Geometry: final body of the model. Coordinates: model frame, mm. A direction names the side the tool comes from. Give positions to 0.01 mm unless a question says otherwise; leave off trailing zeros. Loops run counter-clockwise (first coordinate to the right, second up) from the corner with the lowest first, then second, coordinate; pieces in that order, holes last.
from build123d import *

# Parameters (mm, degrees)
F1_DEPTH  = 22.352
F2_DEPTH  = 3.175
F3_R      = 10.922
F5_DEPTH  = 9.652
F6_DEPTH  = 25.4
F7_R      = 3.175
F9_DEPTH  = 9.652
F8_R      = 6.35
F10_DEPTH = 3.175


with BuildPart() as f1:
    # F0 (on Front) → F1 (new body, symmetric)
    with BuildSketch(Plane.XZ):
        Polygon((28.1862923991, 4.826), (2.7862923991, 4.826), (-16.2637076009, 37.8215678842), (-24.6225847982, 32.9955678842), (-2.7862923991, -4.826), (63.5, -4.826), (63.5, 4.826), align=None)
    extrude(amount=F1_DEPTH, both=True)

    # F0 (on Front) → F2 (join, symmetric)
    with BuildSketch(Plane.XZ):
        Polygon((-16.2637076009, 37.8215678842), (2.7862923991, 4.826), (28.1862923991, 4.826), align=None)
    extrude(amount=F2_DEPTH, both=True)

    # F3
    f3_edges = [f1.edges().sort_by_distance(p)[0] for p in [
        (-20.443146, -22.352, 35.408568),
        (-20.443146, 22.352, 35.408568),
    ]]
    fillet(f3_edges, radius=F3_R)

    # F4 (on face) → F5 (join)
    with BuildSketch(Plane.XY.offset(4.826)):
        with BuildLine():
            Line((63.5, -9.652), (63.5, -22.352))
            ThreePointArc((63.5, -22.352), (85.852, 0), (63.5, 22.352))
            Line((63.5, 22.352), (63.5, 9.652))
            Line((63.5, 9.652), (66.2862923991, 9.652))
            ThreePointArc((66.2862923991, 9.652), (75.9382923991, 0), (66.2862923991, -9.652))
            Line((66.2862923991, -9.652), (63.5, -9.652))
        make_face()
    extrude(amount=-F5_DEPTH)

    # F4 (on face) → F6 (cut)
    with BuildSketch(Plane.XY.offset(4.826)):
        with BuildLine():
            Line((40.8862923991, -9.652), (63.5, -9.652))
            Line((63.5, -9.652), (63.5, 9.652))
            Line((63.5, 9.652), (40.8862923991, 9.652))
            ThreePointArc((40.8862923991, 9.652), (31.2342923991, 0), (40.8862923991, -9.652))
        make_face()
    extrude(amount=-F6_DEPTH, mode=Mode.SUBTRACT)

    # F7 (on face) → F9 (cut, through all)
    with BuildSketch(Plane(origin=(-4.1794385987, 0, -2.413), x_dir=(0, -1, 0), z_dir=(-0.8660254038, 0, -0.5))):
        with Locations((11.43, 29.9642923991)):
            Circle(F7_R)
        with BuildLine():
            ThreePointArc((-8.255, 29.9642923991), (-11.43, 33.1392923991), (-14.605, 29.9642923991))
            ThreePointArc((-14.605, 29.9642923991), (-11.43, 26.7892923991), (-8.255, 29.9642923991))
        make_face()
    extrude(amount=-F9_DEPTH, mode=Mode.SUBTRACT)

    # F8 (on face) → F10 (cut)
    with BuildSketch(Plane(origin=(4.1794385987, 0, 2.413), x_dir=(0, 1, 0), z_dir=(0.8660254038, 0, 0.5))):
        with Locations((-11.43, 29.9642923991)):
            Circle(F8_R)
        with Locations((11.43, 29.9642923991)):
            Circle(F8_R)
    extrude(amount=-F10_DEPTH, mode=Mode.SUBTRACT)


solid = f1.part
Item 1: Pin query (flat end, axial travel): pin 1 (2 mm diameter, centred on y = 10, z = 30.5, fed in from +X); pin 2 (1 mm diameter, centred on x = 51, y = -8.5, fed in from +Z); pin 3 (3 mm diameter, centred on x = -13, y = 14, fed in from +Z); pin 4 (10 mm diameter, centred on x = 16, z = 18, fed in from -Y) (3 decimals). Return the tip coordinate at first contact, or that it passes through.
Values follow:
pin 1: stops at x = -15.13
pin 2: passes through
pin 3: stops at z = 34.77
pin 4: stops at y = -3.175
Item 2: Section query A-A on x = 45.5. Return loops of the section in (y, z).
Values follow:
outline: (-22.35, -4.83) - (-9.65, -4.83) - (-9.65, 4.83) - (-22.35, 4.83) - close; (9.65, -4.83) - (22.35, -4.83) - (22.35, 4.83) - (9.65, 4.83) - close
Item 3: Ray query, probe 1 along Y at (x, z) = (47, 2.5); probe 2 along Y at (x, z) = (66.5, 3); probe 3 along Z at (x, y) = (79, 1.5). Return the intervals inside material, ascending.
Values follow:
probe 1: y = -22.35 to -9.65, 9.65 to 22.35
probe 2: y = -22.15 to -9.65, 9.65 to 22.15
probe 3: z = -4.83 to 4.83
Item 4: Set-up query: faces 1 (the face through (-12.186, -8.697, 24.408)), 2 (the face through (6, -3.175, 15)), 3 (the face through (53, -9.652, 0)). Return all of +Z, -Z, +X, -X, +Y, -Y with unobstructed straight access to the full face (end or side cutting, diameter ignored); none if empty.
Values follow:
face 1: none
face 2: +Z, +X, -Y
face 3: +Z, -Z
Item 5: Section query B-B on y = 0. Return loops of the section in (x, z), plus the area to 3 significant figures.
Values follow:
outline: (-24.62, 33) - (-2.79, -4.83) - (31.23, -4.83) - (31.23, 4.83) - (28.19, 4.83) - (-16.26, 37.82) - close; (75.94, -4.83) - (85.85, -4.83) - (85.85, 4.83) - (75.94, 4.83) - close
area: 1,210 mm2
Item 6: Section query C-C on z = 10.5. Return loops of the section in (x, y) (3 decimals).
Values follow:
outline: (-11.635, -22.352) - (-0.49, -22.352) - (-0.49, -3.175) - (20.543, -3.175) - (20.543, 3.175) - (-0.49, 3.175) - (-0.49, 22.352) - (-11.635, 22.352) - close
Item 7: Draft query along Z for faces 4 (the face through (6, 3.175, 15)), 5 (the face through (44, 10, 4.826)), 6 (the face through (-10.23, -16.47, 24.23)). Return one class per face: +Z half, -Z half, draft (parallel to the pull), parting line (faces both ways), or undercut.
Values follow:
face 4: draft
face 5: +Z half
face 6: undercut
Item 8: Section query D-D on x = 70.5. Return loops of the section in (y, z), plus the area to 3 significant figures.
Values follow:
outline: (-21.23, -4.83) - (-8.68, -4.83) - (-8.68, 4.83) - (-21.23, 4.83) - close; (8.68, -4.83) - (21.23, -4.83) - (21.23, 4.83) - (8.68, 4.83) - close
area: 242 mm2
